Input: part model. Units: mm. Frame: model coordinates. A direction names the side the tool comes from. Coordinates: 2 decimals unless noted, no trailing zeros. Write each loop counter-clockwise with the first axis right and the second up, starting at its lowest first coordinate (ties: lowest second). Pieces come first, ordered by that corner, then holes. Notation, with made-up numbers: (-16.75, -33) - (20.25, -33) arc R15 ccw to (20.25, -26) - close; hole circle Ø5 at (4, -5.75). An arc over 180 degrees is marked (long way). One line per question, with ' | ' between items. Start each with the question number.
1) Section query A-A on x = 58. Return loops of the section in (y, z).
2) Line query: line 1 (X direction, y = 19.75, z = -51.5); line 2 (Z direction, x = 115.5, y = 14); line 3 (Z direction, x = 120, y = 13). Output: solid intervals per line, ascending.
3) Section query C-C on x = 33.5. Return loops of the section in (y, z), and give its area (3 significant figures).
4) First-contact query: P1, Ø4.5, axis at y = 21.5, z = -29.5, coming from the -X side; P2, Ø1.5, axis at y = 22, z = -65, coming from the -X side; P3, Ø6, axis at y = 20.5, z = -68, coming from the -X side; P4, Ø5, axis at x = 132, z = -51.5, coming from the -Y side. Flat tips, straight axial feed; report the tip coordinate or a pass-through.
5) Section query B-B on y = 9.25. Give the number of separate pieces and of enclosed holes in the cut face, and give its area (3 significant figures).
6) Section query D-D on z = -67.5. Return loops of the section in (x, y), and give its area (3 significant figures).
7) Reachability of faces 1 (the cylindrical face through (58.651, 12.818, -43.457)), 2 (the cylindrical face through (132, 16, -60)) from +Z, -Z, +X, -X, +Y, -Y: full face, straight path, thin tool, end or side. Return the list, or none.
8) Draft query along X for faces 3 (the cylindrical face through (113.27, 7.5, -51.52)), 4 (the cylindrical face through (28.9, 12.8, -75.1)). Return one class per face: released by +X, released by -X, zero draft, split by the parting line, or undercut.
```python
from build123d import *

# Parameters (mm, degrees)
BOSS_EXTRUDE1_DEPTH = 26
CUT_EXTRUDE1_START  = -20
CUT_EXTRUDE1_DEPTH  = 20
SKETCH3_W           = 17.5
SKETCH3_H           = 17.5
CUT_EXTRUDE2_DEPTH  = 7
FILLET1_R           = 5
HOLE1_D             = 13
HOLE1_DEPTH         = 30
HOLE2_D             = 6.5
HOLE2_DEPTH         = 30
SKETCH8_R           = 10
BOSS_EXTRUDE2_DEPTH = 20
HOLE3_D             = 10
HOLE3_DEPTH         = 30


with BuildPart() as part:
    # Sketch1 → Boss-Extrude1 (new body)
    with BuildSketch(Plane(origin=(0, 0, 0), x_dir=(1, 0, 0), z_dir=(0, 1, 0))):
        with BuildLine():
            Line((0, -25), (140, -25))
            Line((140, -25), (140, 78.289547156))
            ThreePointArc((140, 78.289547156), (128.151891006, 103.027720783), (101.450252951, 109.302865908))
            ThreePointArc((101.450252951, 109.302865908), (28.006457847, 74.395778776), (-22.580645161, 10.729140884))
            ThreePointArc((-22.580645161, 10.729140884), (-21.13325013, -13.356112419), (0, -25))
        make_face()
    extrude(amount=BOSS_EXTRUDE1_DEPTH)

    # Sketch2 → Cut-Extrude1 (cut)
    with BuildSketch(Plane(origin=(0, 26, 0), x_dir=(1, 0, 0), z_dir=(0, 1, 0)).offset(CUT_EXTRUDE1_START)):
        with BuildLine():
            Line((88, -18), (88, 7))
            Line((88, 7), (114.7, 7))
            Line((114.7, 7), (114.7, 20))
            Line((114.7, 20), (133, 20))
            Line((133, 20), (133, 45))
            Line((133, 45), (114.7, 45))
            Line((114.7, 45), (114.7, 58))
            Line((114.7, 58), (133, 58))
            Line((133, 58), (133, 78.289547156))
            ThreePointArc((133, 78.289547156), (123.764072516, 97.573635258), (102.949409781, 102.465283821))
            ThreePointArc((102.949409781, 102.465283821), (39.68753142, 74.427574639), (-7.525899138, 23.840319674))
            ThreePointArc((-7.525899138, 23.840319674), (21.489023757, 12.775831009), (17.349351573, -18))
            Line((17.349351573, -18), (88, -18))
        make_face()
    extrude(amount=CUT_EXTRUDE1_DEPTH, mode=Mode.SUBTRACT)

    # Sketch3 → Cut-Extrude2 (cut)
    with BuildSketch(Plane(origin=(0, 26, 0), x_dir=(1, 0, 0), z_dir=(0, 1, 0))):
        with Locations((124.25, -9.25)):
            Rectangle(SKETCH3_W, SKETCH3_H)
    extrude(amount=-CUT_EXTRUDE2_DEPTH, mode=Mode.SUBTRACT)

    # Fillet1
    fillet1_edges = [part.edges().sort_by_distance(p)[0] for p in [
        (123.85, 6, -58),
        (115.5, 22.5, 18),
        (115.5, 22.5, 0.5),
        (133, 22.5, 0.5),
        (133, 22.5, 18),
        (88, 16, 18),
        (133, 16, -45),
        (133, 16, -20),
        (114.7, 16, -20),
        (114.7, 16, -7),
        (88, 16, -7),
        (114.7, 16, -58),
        (133, 16, -58),
        (114.7, 16, -45),
        (-7.525899138, 16, -23.840319674),
        (17.349351573, 16, 18),
        (52.674675786, 6, 18),
        (88, 6, 5.5),
        (101.35, 6, -7),
        (114.7, 6, -13.5),
        (123.85, 6, -20),
        (133, 6, -32.5),
        (123.85, 6, -45),
        (114.7, 6, -51.5),
        (21.489023757, 6, -12.775831009),
    ]]
    fillet(fillet1_edges, radius=FILLET1_R)

    # Hole1
    with Locations(Plane(origin=(0, 26, 0), x_dir=(1, 0, 0), z_dir=(0, 1, 0))):
        with Locations((0, 0)):
            Hole(HOLE1_D / 2, depth=HOLE1_DEPTH)

    # Hole2
    with Locations(Plane(origin=(0, 26, 0), x_dir=(1, 0, 0), z_dir=(0, 1, 0))):
        with Locations((120, 51.5), (132, 51.5), (120, 13.5), (132, 13.5)):
            Hole(HOLE2_D / 2, depth=HOLE2_DEPTH)

    # Sketch8 → Boss-Extrude2 (add)
    with BuildSketch(Plane(origin=(0, 6, 0), x_dir=(1, 0, 0), z_dir=(0, 1, 0))):
        with Locations(Location((58, 38.5, 0), (0, 0, 270))):
            Circle(SKETCH8_R)
    extrude(amount=BOSS_EXTRUDE2_DEPTH)

    # Hole3
    with Locations(Plane(origin=(0, 26, 0), x_dir=(1, 0, 0), z_dir=(0, 1, 0))):
        with Locations((58, 38.5)):
            Hole(HOLE3_D / 2, depth=HOLE3_DEPTH)


solid = part.part
```
Answer key:
1) outline: (0, -93.72) - (26, -93.72) - (26, -85.81) - (6, -85.81) - (6, -48.5) - (26, -48.5) - (26, -43.5) - (0, -43.5) - close; (0, -33.5) - (26, -33.5) - (26, -28.5) - (6, -28.5) - (6, 13) arc R5 cw to (11, 18) - (26, 18) - (26, 25) - (0, 25) - close
2) line 1: 4.09 to 13.51, 114.7 to 116.75, 123.25 to 128.75, 135.25 to 140 | line 2: -109.2 to -101.95, -55.71 to -47.29, -17.71 to 25 | line 3: -107.79 to -100.07, -58 to -54.75, -48.25 to -45, -20 to -16.75, -10.25 to 25
3) outline: (0, -78.59) - (26, -78.59) - (26, -69.81) - (6, -69.81) - (6, 13) arc R5 cw to (11, 18) - (26, 18) - (26, 25) - (0, 25) - close | area: 943 mm²
4) P1: x = -13.65 | P2: x = 16.31 | P3: x = 17.11 | P4: through
5) separate pieces: 2 | enclosed holes: 7 | area: 6,620 mm²
6) outline: (19.84, 0) - (140, 0) - (140, 26) - (133, 26) - (133, 6) - (30.6, 6) - (30.6, 26) - (19.84, 26) - close | area: 1,080 mm²
7) face 1: +Y, -Y | face 2: +Y
8) face 3: undercut | face 4: released by -X
